Part model, mm, in its own coordinate system. A direction names the side the tool comes from. Round coordinates to 2 decimals unless told otherwise and drop trailing zeros. Loops run counter-clockwise (first coordinate to the right, second up) from the corner with the lowest first, then second, coordinate; pieces in that order, holes last. Notation, with made-up numbers: M 54.25,-11.75 L 110.25,-11.75 A10 ccw 110.25,2.25 Z; hole C 0,18 d10. An arc over 180 degrees is marked long. Put each result on its own line as item: value. Start each with the question number.
```python
from build123d import *

# Parameters (mm, degrees)
SKETCH1_W           = 76.2
SKETCH1_H           = 63.5
BOSS_EXTRUDE1_DEPTH = 2.54
SKETCH2_W           = 76.2
SKETCH2_H           = 6.75
BOSS_EXTRUDE2_DEPTH = 4
SKETCH3_R           = 2.032
CUT_EXTRUDE1_DEPTH  = 3.81
SKETCH4_R           = 15
CUT_EXTRUDE2_DEPTH  = 10


with BuildPart() as part:
    # Sketch1 → Boss-Extrude1 (new body)
    with BuildSketch(Plane.XY):
        with Locations((38.1, 31.75)):
            Rectangle(SKETCH1_W, SKETCH1_H)
    extrude(amount=BOSS_EXTRUDE1_DEPTH)

    # Sketch2 → Boss-Extrude2 (add)
    with BuildSketch(Plane(origin=(0, 0, 0), x_dir=(-1, 0, 0), z_dir=(0, 0, -1))):
        with Locations((-38.1, 60.125)):
            Rectangle(SKETCH2_W, SKETCH2_H)
        with Locations((-38.1, 3.375)):
            Rectangle(SKETCH2_W, SKETCH2_H)
    extrude(amount=BOSS_EXTRUDE2_DEPTH)

    # Sketch3 → Cut-Extrude1 (cut)
    with BuildSketch(Plane(origin=(0, 0, -4), x_dir=(-1, 0, 0), z_dir=(0, 0, -1))):
        with Locations((-63.5, 60.125)):
            Circle(SKETCH3_R)
        with Locations((-63.5, 3.375)):
            Circle(SKETCH3_R)
        with Locations((-12.7, 3.375)):
            Circle(SKETCH3_R)
        with Locations((-12.7, 60.125)):
            Circle(SKETCH3_R)
    extrude(amount=-CUT_EXTRUDE1_DEPTH, mode=Mode.SUBTRACT)

    # Sketch4 → Cut-Extrude2 (cut)
    with BuildSketch(Plane.XY.offset(2.54)):
        with Locations((38.1, 31.75)):
            Circle(SKETCH4_R)
    extrude(amount=-CUT_EXTRUDE2_DEPTH, mode=Mode.SUBTRACT)


solid = part.part
```
1. Wall check: L1, parallel to Y at x = 12.7, z = -3.05; L2, parallel to Y at x = 38.1, z = 1.45; L3, parallel to Y at x = 24.5, z = -1.5. Give the ranges that are in metal, low to high.
2. Cut at B-B, the plane y = 31.75. Give the cut face in (x, z).
3. Cut at C-C, the plane x = 38.1. Give the cut face in (y, z), and give its area (3 significant figures).
4. Drop flat-ended pins along their axis: pin 1 (1.2 mm diameter, centred on x = 13.5, y = 61, fed in from -Z); pin 2 (25 mm diameter, centred on x = 43, y = 29.5, fed in from -Z). Give the stop position or say it passes through.
5. Cut at A-A, the plane z = -1. Give the cut face in (x, y) (3 decimals), and give its area (3 significant figures).
6. Mould opens along Y. For faces 4 (the flat face through (39, 60, -4)), 5 (the cylindrical face through (14.198, 61.498, -2.122)), 6 (the flat face through (39, 63.5, -1)) say: released by +Y, released by -Y, zero draft, split by the parting line, or undercut.
7. Which spindle directions (+Z, -Z, +X, -X, +Y, -Y) get a long thin tool onto all of the face, cutting with end or side? Do faces 1 (the cylindrical face through (64.998, 61.498, -2.122)), 2 (the flat face through (0, 31, 1)), 3 (the flat face through (39, 56.75, -2)). Say none if no direction does.
8. Cut at D-D, the plane x = 21.5. Give the cut face in (y, z).
Results list:
1. L1: y = 0 to 1.34, 5.41 to 6.75, 56.75 to 58.09, 62.16 to 63.5
1. L2: y = 0 to 16.75, 46.75 to 63.5
1. L3: y = 0 to 6.75, 56.75 to 63.5
2. outline: M 0,0 L 23.1,0 L 23.1,2.54 L 0,2.54 Z; M 53.1,0 L 76.2,0 L 76.2,2.54 L 53.1,2.54 Z
3. outline: M 0,-4 L 6.75,-4 L 6.75,0 L 16.75,0 L 16.75,2.54 L 0,2.54 Z; M 46.75,0 L 56.75,0 L 56.75,-4 L 63.5,-4 L 63.5,2.54 L 46.75,2.54 Z
3. area: 139 mm^2
4. pin 1: stops at z = -0.19
4. pin 2: stops at z = 0
5. outline: M 0,0 L 76.2,0 L 76.2,6.75 L 0,6.75 Z; M 0,56.75 L 76.2,56.75 L 76.2,63.5 L 0,63.5 Z; hole C 12.7,3.375 d4.064; hole C 12.7,60.125 d4.064; hole C 63.5,3.375 d4.064; hole C 63.5,60.125 d4.064
5. area: 977 mm^2
6. face 4: zero draft
6. face 5: undercut
6. face 6: released by +Y
7. face 1: -Z
7. face 2: +Z, -Z, -X, +Y, -Y
7. face 3: -Z, +X, -X
8. outline: M 0,-4 L 6.75,-4 L 6.75,0 L 56.75,0 L 56.75,-4 L 63.5,-4 L 63.5,2.54 L 0,2.54 Z
